Here's how the part is built. I have some questions about the finished solid (model axes, mm). A direction names the side the tool comes from. Coordinates: 2 decimals unless noted, no trailing zeros. Loops run counter-clockwise (first coordinate to the right, second up) from the corner with the lowest first, then second, coordinate; pieces in that order, holes last.
Autodesk Inventor part; units mm, degrees
ref_plane "YZ Plane" through (0, 0, 0) normal (1, 0, 0) x (0, 1, 0)
ref_plane "XZ Plane" through (0, 0, 0) normal (0, 1, 0) x (-1, 0, 0)
ref_plane "XY Plane" through (0, 0, 0) normal (0, 0, 1) x (1, 0, 0)
sketch "Sketch1" plane through (0, 0, 0) normal (0, 0, 1) x (1, 0, 0)
  line L0 (0, 0) -> (0, 99.2)
  line L1 (0.9, 0) -> (1.5, 0)
  line L2 (1.5, 0) -> (1.5, 3.2)
  line L3 (1.5, 3.2) -> (2.1, 3.2)
  line L4 (2.1, 3.2) -> (2.1, 22.1)
  line L5 (2.1, 22.1) -> (2.5, 22.1)
  line L6 (2.5, 22.1) -> (2.5, 86.7)
  line L7 (2.5, 86.7) -> (3.1, 87.3)
  line L8 (3.1, 87.3) -> (3.1, 92.7)
  line L9 (3.1, 92.7) -> (2.5, 92.7)
  line L10 (2.5, 92.7) -> (2.5, 99.2)
  line L11 (2.5, 99.2) -> (2.075, 99.2)
  line L12 (2.075, 99.2) -> (2.075, 92.7)
  line L13 (2.075, 92.7) -> (1.9, 92.3)
  line L14 (1.9, 92.3) -> (1.9, 5.2)
  line L15 (1.9, 5.2) -> (0.9, 5.2)
  line L16 (0.9, 5.2) -> (0.9, 0)
  dimension "d0" = 45
  dimension "d1" = 99.2
  dimension "d2" = 92.7
  dimension "d3" = 86.7
  dimension "d4" = 22.1
  dimension "d5" = 3.2
  dimension "d6" = 1.8
  dimension "d7" = 3
  dimension "d8" = 4.2
  dimension "d9" = 5.2
  dimension "d10" = 3.8
  dimension "d11" = 4.15
  dimension "d12" = 5
  dimension "d13" = 6.2
  dimension "d14" = 92.3
  dimension "d15" = 5
revolve "Revolution1" add sketch "Sketch1" angle 360 about axis through (0, 0, 0) along (0, 1, 0)
sketch "Sketch2" plane through (0, 0, 0) normal (0, 0, 1) x (1, 0, 0)
  line L0 (-0.9, 0) -> (0.9, 0)
  line L1 (-4, 96) -> (0, 96) construction
  line L2 (0, -19.84) -> (0, 119.04)
  line L3 (0, 96) -> (-8, 96)
  line L4 (-8, 96) -> (-8, 99.2)
  line L5 (-8, 99.2) -> (0, 99.2)
  line L6 (0, 99.2) -> (0, 96)
  line L7 (-2.075, 99.2) -> (2.075, 99.2)
  dimension "d17" = 96
  dimension "d18" = 4
  dimension "d19" = 8
extrude "Extrusion1" cut sketch "Sketch2" against normal mid plane 2
properties part number "PP-09" material "ABS Plastic"
1. I need wall thicknesses on line 1 along X through (y, z) = (79, 0); line 2 along Z through (x, y) = (0, 96.25) (3 decimals). Which ranges of each line are inside material? Lowest first, please.
2. I want a section at C-C (y = 17.5). Please give me the cut outline in (x, z).
3. On a 3-axis mill with a long thin cutter (end or side, diameter ignored), from which of +Z, -Z, +X, -X, +Y, -Y can I reach the whole of each face in a straight line? I mean faces 1 (the cylindrical face through (2.003, 12.782, -0.631)), 2 (the cylindrical face through (1.92, 95.9, -0.79)), 3 (the cylindrical face through (1.43, 90.04, 2.75)). Say none if no direction works.
4. We'd pull the mould along Z, two halves only. Please class faces 4 (the cylindrical face through (2.385, 95.996, -0.751)), 5 (the flat face through (2, 99.2, 1)), 6 (the cylindrical face through (-1.9, 48.14, 0.08)), 7 (the cylindrical face through (0.86, 2.56, 0.27)): +Z half, -Z half, draft (parallel to the pull), parting line (faces both ways), or undercut.
5. For pin 1 (0.5 mm diameter, centred on x = -2, y = 97.5, fed in from -Z); pin 2 (0.5 mm diameter, centred on x = -2, z = -0.5, fed in from +Y); pin 3 (3 mm diameter, centred on y = 60, z = 1, fed in from +X), each with a flat end and sliding along its axis, tell me the tip position at first contact or that it passes through.
6. I want a section at B-B (y = 79). Please give me the cut outline in (x, z).
Response values:
1. line 1: x = -2.5 to -1.9, 1.9 to 2.5
1. line 2: z = -2.5 to -2.075, 2.075 to 2.5
2. outline: circle Ø4.2 at (0, 0); hole circle Ø3.8 at (0, 0)
3. face 1: -Y
3. face 2: +Y
3. face 3: +Y, -Y
4. face 4: parting line
4. face 5: draft
4. face 6: undercut
4. face 7: undercut
5. pin 1: stops at z = -1.79
5. pin 2: stops at y = 96
5. pin 3: stops at x = 2.5
6. outline: circle Ø5 at (0, 0); hole circle Ø3.8 at (0, 0)
